Geometry check sheet. Reference: the model listing, model coordinates, mm. A direction names the side the tool comes from. Give positions to 0.01 mm unless a question says otherwise; leave off trailing zeros. Order: outer loops, then holes, each group sorted by start corner. A loop starts at its lowest first (then second) coordinate and runs counter-clockwise, first axis right, second up.
```python
from build123d import *
from OCP.BRepAlgoAPI import BRepAlgoAPI_Cut
from OCP.TopTools import TopTools_ListOfShape

# Parameters (mm, degrees)
SCHIZZO1_R                   = 25
SCHIZZO1_R_2                 = 15
ESTRUSIONE_ESTRUSIONE1_DEPTH = 30
ESTRUSIONE_ESTRUSIONE2_DEPTH = 25
TAGLIO_ESTRUSIONE1_DEPTH     = 123.613212991
FORO_18_0_18_1_D             = 18
FORO_18_0_18_1_CSINK_D       = 18.05
FORO_18_0_18_1_CSINK_ANGLE   = 90
FORO_10_0_10_1_D             = 10
FORO_10_0_10_1_CSINK_D       = 10.05
FORO_10_0_10_1_CSINK_ANGLE   = 90
TAGLIO_ESTRUSIONE2_START     = -51
TAGLIO_ESTRUSIONE2_DEPTH     = 51
RACCORDO1_R                  = 5


with BuildPart() as part:
    # Schizzo1 → Estrusione-Estrusione1 (new, symmetric)
    with BuildSketch(Plane.XY):
        Circle(SCHIZZO1_R)
        Circle(SCHIZZO1_R_2, mode=Mode.SUBTRACT)
    extrude(amount=ESTRUSIONE_ESTRUSIONE1_DEPTH, both=True)

    # Schizzo1<6> → Estrusione-Estrusione2 (add, symmetric)
    with BuildSketch(Plane.XY):
        with BuildLine():
            Line((11.5, 45), (-11.5, 45))
            Line((-11.5, 45), (-11.5, 22.19797288))
            ThreePointArc((-11.5, 22.19797288), (12.990381057, 21.360009363), (25, 0))
            ThreePointArc((25, 0), (17.67766953, -17.67766953), (0, -25))
            Line((0, -25), (97, -25))
            Line((97, -25), (97, -9))
            Line((97, -9), (42, -9))
            ThreePointArc((42, -9), (40.585786438, -8.414213562), (40, -7))
            Line((40, -7), (40, 7))
            ThreePointArc((40, 7), (40.585786438, 8.414213562), (42, 9))
            Line((42, 9), (97, 9))
            Line((97, 9), (97, 25))
            Line((97, 25), (11.5, 25))
            Line((11.5, 25), (11.5, 45))
        make_face()
    extrude(amount=ESTRUSIONE_ESTRUSIONE2_DEPTH, both=True)

    # Schizzo3 → Taglio-Estrusione1 (cut, through all)
    with BuildSketch(Plane.XY.offset(30)):
        Polygon((1.5, 45), (-1.5, 45), (-1.5, 14.924811557), (0, 15), (1.5, 14.924811557), align=None)
    extrude(amount=-TAGLIO_ESTRUSIONE1_DEPTH, mode=Mode.SUBTRACT)

    # Foro Ø18.0 (18)-1 (through all)
    with Locations(Plane(origin=(71.999996961, 25, 6.74e-07), x_dir=(1, 0, 0), z_dir=(0, 1, 0))):
        with Locations((0, 0)):
            CounterSinkHole(FORO_18_0_18_1_D / 2, FORO_18_0_18_1_CSINK_D / 2, counter_sink_angle=FORO_18_0_18_1_CSINK_ANGLE)

    # Foro Ø10.0 (10)-1 (through all)
    with Locations(Plane(origin=(-11.5, 35, 15), x_dir=(0, 0, -1), z_dir=(-1, 0, 0))):
        with Locations((0, 0), (30, 0)):
            CounterSinkHole(FORO_10_0_10_1_D / 2, FORO_10_0_10_1_CSINK_D / 2, counter_sink_angle=FORO_10_0_10_1_CSINK_ANGLE)


with BuildPart() as taglio_estrusione2_tool:
    # Taglio-Estrusione2: read off the stored shape, not the designer's step
    # Taglio-Estrusione2 outline → Taglio-Estrusione2 (new body)
    with BuildSketch(Plane(origin=(0, 25, 0), x_dir=(1, 0, 0), z_dir=(0, 1, 0)).offset(TAGLIO_ESTRUSIONE2_START)):
        with BuildLine():
            Line((97, 25), (71.999996961, 25))
            ThreePointArc((71.999996961, 25), (89.677666491, 17.67766953), (96.999996961, 0))
            Line((96.999996961, 0), (97, 25))
        make_face()
        with BuildLine():
            Line((97, -25), (96.999996961, 0))
            ThreePointArc((96.999996961, 0), (89.677666491, -17.67766953), (71.999996961, -25))
            Line((71.999996961, -25), (97, -25))
        make_face()
    extrude(amount=TAGLIO_ESTRUSIONE2_DEPTH)


with BuildPart() as part_1:
    add(part.part)

    # Taglio-Estrusione2: cut by taglio_estrusione2_tool, with a tolerance
    taglio_estrusione2_stock = TopTools_ListOfShape()
    taglio_estrusione2_stock.Append(part_1.part.wrapped)
    taglio_estrusione2_tools = TopTools_ListOfShape()
    taglio_estrusione2_tools.Append(taglio_estrusione2_tool.part.wrapped)
    taglio_estrusione2_cut = BRepAlgoAPI_Cut()
    taglio_estrusione2_cut.SetArguments(taglio_estrusione2_stock)
    taglio_estrusione2_cut.SetTools(taglio_estrusione2_tools)
    taglio_estrusione2_cut.SetFuzzyValue(0.00001)
    taglio_estrusione2_cut.Build()
    add(Compound.cast(taglio_estrusione2_cut.Shape()).solids(), mode=Mode.REPLACE)

    # Raccordo1
    raccordo1_edges = [part_1.edges().sort_by_distance(p)[0] for p in [
        (-6.5, 45, 25),
        (-6.5, 45, -25),
        (6.5, 45, -25),
        (6.5, 45, 25),
    ]]
    fillet(raccordo1_edges, radius=RACCORDO1_R)


solid = part_1.part
```
Q1. Cross-section at D-D, the plane x = -3. Record the boundary of the cut face in (y, z), and give its area (3 significant figures).
Q2. Release check for a two-part mould opening along Y. For faces 1 (the face through (48, -25, 0)), 2 (the face through (-6.42, 39.88, -16.08)), 3 (the face through (-11.5, 34, 0)) record: pulls with the +Y half, pulls with the -Y half, needs draft (parallel to the pull), parting line crosses it, or undercut.
Q3. Cross-section at B-B, the plane z = 15. Record the boundary of the cut face in (x, y) (3 decimals), and give its area (3 significant figures).
Q4. Access from +Z, -Z, +X, -X, +Y, -Y to the whole of each face (thin tool, end or side, straight path). Record for faces 4 (the face through (55, 25, 0)), 5 (the face through (-0.639, -14.986, -0.42)), 6 (the face through (40, 0, 0)), 7 (the face through (-1.5, 30, 0)).
Q5. Gauge pin test, flat ends, axial feed: P1, Ø10, axis at x = 23, y = 21.5, coming from the +Z side; P2, Ø10, axis at y = 39.5, z = 0, coming from the +X side; P3, Ø4, axis at x = 54.5, y = -11, coming from the -Z side. Record the tip position at first contact, or that the pin passes through.
Q6. Thickness scan on L1, parallel to Z at x = 6.5, y = 35; L2, parallel to X at y = 26, z = -24; L3, parallel to Y at x = 60.5, z = 12. Record the ranges inside material, lowest first.
Q7. Cross-section at A-A, the plane y = 35. Record the boundary of the cut face in (x, z) (3 decimals), and give its area (3 significant figures).
Q8. Cross-section at C-C, the plane y = 0. Record the boundary of the cut face in (x, z), and give its area (3 significant figures).
Answers follow:
1. outline: (-24.82, -30) - (-14.7, -30) - (-14.7, 30) - (-24.82, 30) - close; (14.7, -30) - (24.82, -30) - (24.82, -25) - (40, -25) arc R5 ccw to (45, -20) - (45, 20) arc R5 ccw to (40, 25) - (24.82, 25) - (24.82, 30) - (14.7, 30) - close; hole circle Ø10 at (35, -15); hole circle Ø10 at (35, 15)
1. area: 2,060 mm2
2. face 1: pulls with the -Y half
2. face 2: undercut
2. face 3: needs draft
3. outline: (-11.5, 22.198) arc R25 ccw to (0, -25) - (92, -25) - (92, -9) - (42, -9) arc R2 cw to (40, -7) - (40, 7) arc R2 cw to (42, 9) - (92, 9) - (92, 25) - (11.5, 25) - (11.5, 30) - (1.5, 30) - (1.5, 14.925) arc R15 cw (long way) to (-1.5, 14.925) - (-1.5, 30) - (-11.475, 30) - (-11.5, 29.975) - close; (-11.5, 40.025) - (-11.475, 40) - (-1.5, 40) - (-1.5, 45) - (-11.5, 45) - close; (1.5, 40) - (11.5, 40) - (11.5, 45) - (1.5, 45) - close
3. area: 4,120 mm2
4. face 4: +Z, -Z, +X, +Y
4. face 5: +Z, -Z
4. face 6: +Z, -Z, +X
4. face 7: +Z, -Z, +Y
5. P1: stops at z = 25
5. P2: stops at x = 11.5
5. P3: stops at z = -25
6. L1: z = -25 to -20, -10 to 10, 20 to 25
6. L2: x = -11.5 to -1.5, 1.5 to 11.5
6. L3: y = -25 to -9, 9 to 25
7. outline: (-11.5, -25) - (-1.5, -25) - (-1.5, -20) - (-11.475, -20) - (-11.5, -20.025) - close; (-11.5, -9.975) - (-11.475, -10) - (-1.5, -10) - (-1.5, 10) - (-11.475, 10) - (-11.5, 9.975) - close; (-11.5, 20.025) - (-11.475, 20) - (-1.5, 20) - (-1.5, 25) - (-11.5, 25) - close; (1.5, -25) - (11.5, -25) - (11.5, -20) - (1.5, -20) - close; (1.5, -10) - (11.5, -10) - (11.5, 10) - (1.5, 10) - close; (1.5, 20) - (11.5, 20) - (11.5, 25) - (1.5, 25) - close
7. area: 600 mm2
8. outline: (-25, -30) - (-15, -30) - (-15, 30) - (-25, 30) - close; (15, -30) - (25, -30) - (25, -25) - (40, -25) - (40, 25) - (25, 25) - (25, 30) - (15, 30) - close
8. area: 1,950 mm2
